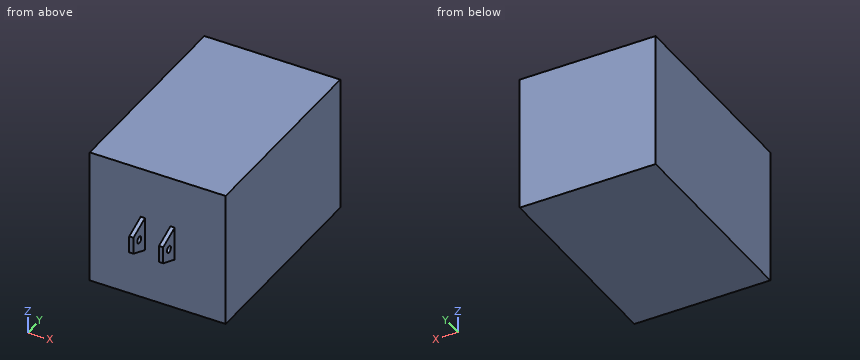
from build123d import *

# Parameters (mm, degrees)
SKETCH1_W           = 40
SKETCH1_H           = 40
BOSS_EXTRUDE1_DEPTH = 60
SKETCH3_R           = 1
BOSS_EXTRUDE2_DEPTH = 5
SKETCH4_W           = 19.244231552
SKETCH4_H           = 7.397169782
CUT_EXTRUDE1_DEPTH  = 3.75


with BuildPart() as part:
    # Sketch1 → Boss-Extrude1 (new body)
    with BuildSketch(Plane(origin=(0, 0, 0), x_dir=(1, 0, 0), z_dir=(0, 1, 0))):
        Rectangle(SKETCH1_W, SKETCH1_H)
    extrude(amount=BOSS_EXTRUDE1_DEPTH)

    # Sketch3 → Boss-Extrude2 (add, symmetric)
    with BuildSketch(Plane(origin=(0, 0, 0), x_dir=(0, 0, -1), z_dir=(1, 0, 0))):
        Polygon((-5, 0), (-2.5, -6), (2.5, -6), (5, 0), align=None)
        with Locations((0, -3)):
            Circle(SKETCH3_R, mode=Mode.SUBTRACT)
    extrude(amount=BOSS_EXTRUDE2_DEPTH, both=True)

    # Sketch4 → Cut-Extrude1 (cut, symmetric)
    with BuildSketch(Plane(origin=(0, 0, 0), x_dir=(0, 0, -1), z_dir=(1, 0, 0))):
        with Locations((0.530352838, -3.698584891)):
            Rectangle(SKETCH4_W, SKETCH4_H)
    extrude(amount=CUT_EXTRUDE1_DEPTH, both=True, mode=Mode.SUBTRACT)


solid = part.part
Can you work these out from the model? Positions are in its coordinate system, mm. Coordinates: 2 decimals unless noted, no trailing zeros. Write each loop counter-clockwise with the first axis right and the second up, starting at its lowest first coordinate (ties: lowest second). Pieces come first, ordered by that corner, then holes. Notation, with made-up numbers: (54, -35) -> (109, -35) arc R18 ccw to (109, -7) -> close; hole circle Ø10 at (46, -12). An arc over 180 degrees is marked (long way). Write each question's results on one line, items separated by ' | '. Start each with the question number.
Item 1: If we section it at A-A, the plane y = -3: Write out the boundary of the cut face in (x, z).
Item 2: Please list where these lines run through material, in increasing order: probe 1 along Z at (x, y) = (4.1, -3); probe 2 along Y at (x, z) = (-4, 0); probe 3 along Y at (x, z) = (-4, 10.5).
Item 3: If we section it at B-B, the plane z = 0: Write out the boundary of the cut face in (x, y), and give its area (3 significant figures).
Item 4: If we section it at D-D, the plane x = -10: Write out the boundary of the cut face in (y, z).
Item 5: I'm going to push flat-ended pins straight in: P1, Ø3, axis at y = -4, z = 0, coming from the +X side; P2, Ø2.5, axis at y = -3, z = 0, coming from the -X side; P3, Ø6, axis at x = 9, z = -12, coming from the -Y side. Where does each tip first touch, or does it pass through?
Item 6: If we section it at C-C, the plane z = -6.5: Write out the boundary of the cut face in (x, y), and give its area (3 significant figures).
Answer block:
1) outline: (-5, -3.75) -> (-3.75, -3.75) -> (-3.75, -1) -> (-5, -1) -> close; (-5, 1) -> (-3.75, 1) -> (-3.75, 3.75) -> (-5, 3.75) -> close; (3.75, -3.75) -> (5, -3.75) -> (5, -1) -> (3.75, -1) -> close; (3.75, 1) -> (5, 1) -> (5, 3.75) -> (3.75, 3.75) -> close
2) probe 1: -3.75 to -1, 1 to 3.75 | probe 2: -6 to -4, -2 to 60 | probe 3: 0 to 60
3) outline: (-20, 0) -> (-5, 0) -> (-5, -2) -> (-3.75, -2) -> (-3.75, 0) -> (3.75, 0) -> (3.75, -2) -> (5, -2) -> (5, 0) -> (20, 0) -> (20, 60) -> (-20, 60) -> close; (-5, -6) -> (-3.75, -6) -> (-3.75, -4) -> (-5, -4) -> close; (3.75, -6) -> (5, -6) -> (5, -4) -> (3.75, -4) -> close | area: 2,410 mm²
4) outline: (0, -20) -> (60, -20) -> (60, 20) -> (0, 20) -> close
5) P1: x = 5 | P2: x = -5 | P3: y = 0
6) outline: (-20, 0) -> (20, 0) -> (20, 60) -> (-20, 60) -> close | area: 2,400 mm²
